Geometry: final body of the model. Coordinates: model frame, mm. Round coordinates to 2 decimals unless told otherwise and drop trailing zeros. Order: outer loops, then holes, each group sorted by start corner. A loop starts at its lowest first (then second) coordinate and runs counter-clockwise, first axis right, second up. Notation, with made-up numbers: (-3, 11.5) -> (7, 11.5) arc R28 ccw to (7, 32.5) -> close; hole circle Ø8 at (-21.75, 83.25). An arc over 180 degrees is marked (long way). Put each result on its own line as item: value.
```python
from build123d import *

# Parameters (mm, degrees)
SKETCH_1_W      = 25
SKETCH_1_H      = 10
SKETCH_1_R      = 1.35
EXTRUDE_1_DEPTH = 2
SKETCH_3_R      = 1.35
EXTRUDE_2_DEPTH = 2
FILLET_2_R      = 40
FILLET_2_R_2    = 20
FILLET_2_R_3    = 30
FILLET_4_R      = 2


with BuildPart() as part:
    # 草图1 → 凸台-拉伸1 (new body)
    with BuildSketch(Plane(origin=(0, 0, 0), x_dir=(1, 0, 0), z_dir=(0, 1, 0))):
        Rectangle(SKETCH_1_W, SKETCH_1_H)
        with Locations(Location((8, 0, 0), (0, 0, 270))):
            Circle(SKETCH_1_R, mode=Mode.SUBTRACT)
        with Locations(Location((-8, 0, 0), (0, 0, 270))):
            Circle(SKETCH_1_R, mode=Mode.SUBTRACT)
    extrude(amount=EXTRUDE_1_DEPTH)

    # 草图3 → 凸台-拉伸2 (add)
    with BuildSketch(Plane(origin=(0, 2, 0), x_dir=(1, 0, 0), z_dir=(0, 1, 0))):
        with BuildLine():
            Line((-12.5, 5), (-12.5, -5))
            ThreePointArc((-12.5, -5), (-62.017500377, -37.077584126), (-46.5, -94))
            Line((-46.5, -94), (-46.5, -153))
            Line((-46.5, -153), (-61.5, -153))
            Line((-61.5, -153), (-61.5, -94))
            ThreePointArc((-61.5, -94), (-67.320253247, -29.493005969), (-12.5, 5))
        make_face()
        with Locations(Location((-54, -149, 0), (0, 0, 270))):
            Circle(SKETCH_3_R, mode=Mode.SUBTRACT)
        with Locations(Location((-63.522724498, -79.241972734, 0), (0, 0, 270))):
            Circle(SKETCH_3_R, mode=Mode.SUBTRACT)
        with Locations(Location((-47.401976264, -11.491855125, 0), (0, 0, 270))):
            Circle(SKETCH_3_R, mode=Mode.SUBTRACT)
        with Locations(Location((-69.309761535, -54.920989975, 0), (0, 0, 270))):
            Circle(SKETCH_3_R, mode=Mode.SUBTRACT)
        with Locations(Location((-63.522724498, -30.600007217, 0), (0, 0, 270))):
            Circle(SKETCH_3_R, mode=Mode.SUBTRACT)
        with Locations(Location((-54, -143, 0), (0, 0, 270))):
            Circle(SKETCH_3_R, mode=Mode.SUBTRACT)
        with Locations(Location((-54, -137, 0), (0, 0, 270))):
            Circle(SKETCH_3_R, mode=Mode.SUBTRACT)
        with Locations(Location((-54, -131, 0), (0, 0, 270))):
            Circle(SKETCH_3_R, mode=Mode.SUBTRACT)
        with Locations(Location((-54, -125, 0), (0, 0, 270))):
            Circle(SKETCH_3_R, mode=Mode.SUBTRACT)
    extrude(amount=-EXTRUDE_2_DEPTH)

    # 圆角2
    # the kernel refuses this fillet: 40, 30, 20 mm, written as the material it adds along each edge
    with BuildSketch(Plane(origin=(-61.5, 2, 94), x_dir=(0, 0, 1), z_dir=(0, -1, 0))) as fillet_2_piece_1:
        with BuildLine():
            CenterArc((11.468694882, 40), FILLET_2_R, 241.625850179, 28.374149821)
            ThreePointArc((-7.540396677, 4.805477158), (-3.683456175, 2.538847918), (0, 0))
            Line((0, 0), (11.468694882, 0))
        make_face()
    extrude(amount=2)
    # the kernel refuses this fillet: 40, 30, 20 mm, written as the material it takes off along each edge
    with BuildSketch(Plane(origin=(-46.5, 23.664306304, 94), x_dir=(-0.733794554453268, 0, -0.6793714387981952), z_dir=(0, -1, 0))) as fillet_2_2_piece_1:
        with BuildLine():
            CenterArc((8.788646711, -19.946288773), FILLET_2_R_2, 94.200030188, 43.005425253)
            Line((-5.887244378, -6.358859997), (0, 0))
            ThreePointArc((0, 0), (3.66193613, -0.134278068), (7.323872259, 0))
        make_face()
    extrude(amount=45.328612608, mode=Mode.SUBTRACT)
    with BuildSketch(Plane(origin=(-12.5, -2.4014787, 5), x_dir=(1, 0, 0), z_dir=(0, 1, 0))) as fillet_2_2_piece_2:
        with BuildLine():
            CenterArc((0.96059148, 40), FILLET_2_R, 267.599016081, 2.400983919)
            ThreePointArc((-0.715120971, 0.035115567), (-0.357497629, 0.018837835), (0, 0))
            Line((0, 0), (0.96059148, 0))
        make_face()
    extrude(amount=6.8029574, mode=Mode.SUBTRACT)
    with BuildSketch(Plane(origin=(-12.5, -0.73103436, -5), x_dir=(1, 0, 0), z_dir=(0, 1, 0))) as fillet_2_2_piece_3:
        with BuildLine():
            CenterArc((0.210076235, -30), FILLET_2_R_3, 90, 0.959672209)
            ThreePointArc((-0.292383464, -0.004208058), (-0.146194213, -0.001931656), (0, 0))
            Line((0, 0), (0.210076235, 0))
        make_face()
    extrude(amount=3.462068721, mode=Mode.SUBTRACT)

    # 圆角4
    fillet_4_edges = [part.edges().sort_by_distance(p)[0] for p in [
        (12.5, 1, 5),
        (12.5, 1, -5),
    ]]
    fillet(fillet_4_edges, radius=FILLET_4_R)


solid = part.part
```
1. Cut plane B-B on x = -4. Return loops of the section in (y, z), and give its area (3 significant figures).
Ans:
outline: (0, -5) -> (2, -5) -> (2, 5) -> (0, 5) -> close
area: 20.0 mm²
2. Material intervals for probe 1 along X at (y, z) = (1.1, 131); probe 2 along Z at (x, y) = (-1, 0.4); probe 3 along X at (y, z) = (1.5, 130), sorted ascending.
Ans:
probe 1: -61.5 to -55.35, -52.65 to -46.5
probe 2: -5 to 5
probe 3: -61.5 to -54.91, -53.09 to -46.5
3. Cut plane A-A on y = 1.25. State how many separate pieces and enclosed holes the cut face has, and give its area (3 significant figures).
Ans:
separate pieces: 1
enclosed holes: 11
area: 2,220 mm²
4. Draft query along Z for faces 1 (the face through (-62.754, 1.014, 95.531)), 2 (the face through (-63, 0, 74)), 3 (the face through (-47.93, 1.01, 95.24)). Return one class per face: +Z half, -Z half, draft (parallel to the pull), parting line (faces both ways), or undercut.
Ans:
face 1: +Z half
face 2: draft
face 3: undercut
5. Contact query for flat-ended pins moving along their axis: P1, Ø0.6, axis at y = 1, z = 127, coming from the -X side; P2, Ø2, axis at x = -54, z = 137, coming from the +Y side. Output: stop coordinate, or through.
Ans:
P1: x = -61.5
P2: through
6. Cut plane C-C on z = 71. Return loops of the section in (x, y).
Ans:
outline: (-72.15, 0) -> (-62.65, 0) -> (-62.65, 2) -> (-72.15, 2) -> close
